Geometry check sheet. Reference: drawing and pictorial views, mm from the part's lowest x, y, z. A direction names the side the tool comes from. Round coordinates to 2 decimals unless told otherwise and drop trailing zeros. Order: outer loops, then holes, each group sorted by start corner. A loop starts at its lowest first (then second) coordinate and runs counter-clockwise, first axis right, second up.
(1) Sectioned sample at C-C (z = 116). Record the boundary of the cut face in (x, y), plus the area to 3 significant figures.
(2) Set-up check for the marked faces 1 and 2: record each of +Z, -Z, +X, -X, +Y, -Y from which the full face is reachable in a straight line by a thin tool's end or side.
(3) Sectioned sample at D-D (z = 17.5). Record the boundary of the cut face in (x, y).
(4) Sectioned sample at A-A (x = 31). Record the boundary of the cut face in (y, z).
(5) Material ranges on line 1 along X through (y, z) = (30, 39.5); line 2 along Z through (x, y) = (14.5, 38.5); line 3 along Z through (x, y) = (21, 20.5), recorded low to high.
(6) Go/stop test with flat-tipped pins: pin 1 (2 mm diameter, centred on y = 54.5, z = 42.5, fed in from -X); pin 2 (12 mm diameter, centred on x = 54.5, z = 56.5, fed in from +Y); pin 3 (3 mm diameter, centred on y = 38.5, z = 76, fed in from +X). Record where each tip stops, or that it passes through.
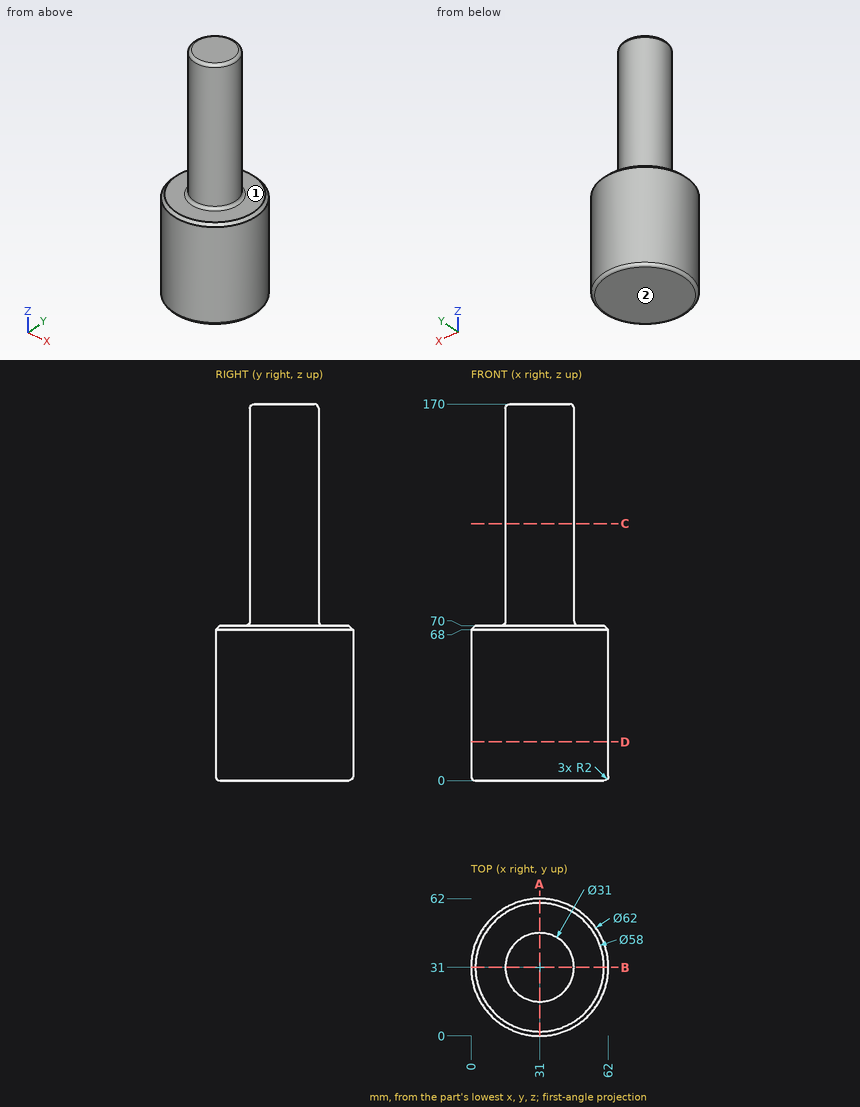
Answer below:
1. outline: circle Ø31 at (31, 31)
1. area: 755 mm2
2. face 1: +Z
2. face 2: -Z, +X, -X, +Y, -Y
3. outline: circle Ø62 at (31, 31)
4. outline: (0, 2) arc R2 ccw to (2, 0) - (60, 0) arc R2 ccw to (62, 2) - (62, 68) - (60, 70) - (48.5, 70) arc R2 cw to (46.5, 72) - (46.5, 168) arc R2 ccw to (44.5, 170) - (17.5, 170) arc R2 ccw to (15.5, 168) - (15.5, 72) arc R2 cw to (13.5, 70) - (2, 70) - (0, 68) - close
5. line 1: x = 0.02 to 61.98
5. line 2: z = 0 to 70
5. line 3: z = 0 to 169.73
6. pin 1: stops at x = 9.68
6. pin 2: stops at y = 56.59
6. pin 3: stops at x = 45.29
